```python
from build123d import *

# Parameters (mm, degrees)
SKETCH1_W                      = 25.4
SKETCH1_H                      = 31.75
BOSS_EXTRUDE1_DEPTH            = 41.275
SKETCH2_R                      = 3.175
F_1_4_THROUGH_HOLE_DEPTH       = 51.998051433
SKETCH3_R                      = 1.984375
F_10_32_THREADED_HOLES_1_DEPTH = 25.4


with BuildPart() as part:
    # Sketch1 → Boss-Extrude1 (new body)
    with BuildSketch(Plane(origin=(0, 0, 0), x_dir=(1, 0, 0), z_dir=(0, 1, 0))):
        Rectangle(SKETCH1_W, SKETCH1_H)
    extrude(amount=BOSS_EXTRUDE1_DEPTH)

    # Sketch2 → 1/4" Through Hole (cut, through all)
    with BuildSketch(Plane(origin=(12.7, 0, 0), x_dir=(0, 0, -1), z_dir=(1, 0, 0))):
        with Locations((0, 9.525)):
            Circle(SKETCH2_R)
    extrude(amount=-F_1_4_THROUGH_HOLE_DEPTH, mode=Mode.SUBTRACT)

    # Sketch3 → 10-32 Threaded Holes (1") (cut)
    with BuildSketch(Plane(origin=(0, 41.275, 0), x_dir=(1, 0, 0), z_dir=(0, 1, 0))):
        with Locations(Location((0, 6.35, 0), (0, 0, 270))):
            Circle(SKETCH3_R)
        with Locations(Location((0, -6.35, 0), (0, 0, 270))):
            Circle(SKETCH3_R)
    extrude(amount=-F_10_32_THREADED_HOLES_1_DEPTH, mode=Mode.SUBTRACT)


solid = part.part
```
Input: part model. Units: mm. Frame: model coordinates. A direction names the side the tool comes from. Give positions to 0.01 mm unless a question says otherwise; leave off trailing zeros. Loops run counter-clockwise (first coordinate to the right, second up) from the corner with the lowest first, then second, coordinate; pieces in that order, holes last. Notation, with made-up numbers: M 17,-30.75 L 32,-30.75 A15 cw 32,-8.75 Z; hole C -9,-24.5 d3. An arc over 180 degrees is marked long. Answer as CSV lines item,"result". Start each with the question number.
1. Section D-D on z = 6.35. Return loops of the section in (x, y) (3 decimals), plus the area to 3 significant figures.
2. Section B-B on x = -1.25. Return loops of the section in (y, z) (3 decimals).
3. Pull-direction query (Y, two-part tool) for faces 1 (the face through (0, 15.875, -6)), 2 (the face through (0, 20, 15.875)), 3 (the face through (0, 0, 0)), 4 (the face through (0.18, 12.2, -1.71)); classes: released by +Y, released by -Y, zero draft, split by the parting line, or undercut.
4. Section A-A on z = 0. Return loops of the section in (x, y) (3 decimals).
5. Line query: L1, parallel to Y at x = 9.75, z = 0 (3 decimals); L2, parallel to X at y = 39, z = -6.5; L3, parallel to Z at x = -1, y = 24.5 (3 decimals). Output: solid intervals per line, ascending.
6. Section C-C on y = 37.5. Return loops of the section in (x, z) (3 decimals).
7. Pin query (flat end, axial travel): P1, Ø2, axis at x = 1, z = -7, coming from the +Y side (3 decimals); P2, Ø3, axis at x = 0, z = 6.35, coming from the +Y side (3 decimals). Return the tip coordinate at first contact, or that it passes through.
8. Reachability of faces 5 (the face through (0, 15.875, 6)), 6 (the face through (0, 20, -15.875)) from +Z, -Z, +X, -X, +Y, -Y: full face, straight path, thin tool, end or side. Return the list, or none.
Computed values:
1,outline,"M -12.7,0 L 12.7,0 L 12.7,41.275 L 1.984,41.275 L 1.984,15.875 L -1.984,15.875 L -1.984,41.275 L -12.7,41.275 Z"
1,area,"948 mm²"
2,outline,"M 0,-15.875 L 41.275,-15.875 L 41.275,-7.891 L 15.875,-7.891 L 15.875,-4.809 L 41.275,-4.809 L 41.275,4.809 L 15.875,4.809 L 15.875,7.891 L 41.275,7.891 L 41.275,15.875 L 0,15.875 Z; hole C 9.525,0 d6.35"
3,face 1,"released by +Y"
3,face 2,"zero draft"
3,face 3,"released by -Y"
3,face 4,"undercut"
4,outline,"M -12.7,0 L 12.7,0 L 12.7,6.35 L -12.7,6.35 Z; M -12.7,12.7 L 12.7,12.7 L 12.7,41.275 L -12.7,41.275 Z"
5,L1,"y = 0 to 6.35, 12.7 to 41.275"
5,L2,"x = -12.7 to -1.98, 1.98 to 12.7"
5,L3,"z = -15.875 to -8.064, -4.636 to 4.636, 8.064 to 15.875"
6,outline,"M -12.7,-15.875 L 12.7,-15.875 L 12.7,15.875 L -12.7,15.875 Z; hole C 0,-6.35 d3.969; hole C 0,6.35 d3.969"
7,P1,"stops at y = 41.275"
7,P2,"stops at y = 15.875"
8,face 5,"+Y"
8,face 6,"-Z, +X, -X, +Y, -Y"
